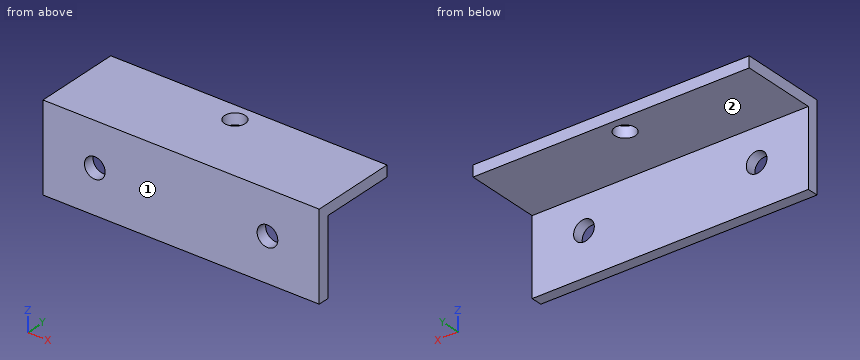
```python
from build123d import *

# Parameters (mm, degrees)
BOSS_EXTRUDE1_DEPTH = 1.6
SKETCH3_W           = 40
SKETCH3_H           = 1.6
BOSS_EXTRUDE3_DEPTH = 11
SKETCH4_R           = 1.5
CUT_EXTRUDE2_DEPTH  = 27.786563796


with BuildPart() as part:
    # Sketch1 → Boss-Extrude1 (new body)
    with BuildSketch(Plane(origin=(0, 0, 0), x_dir=(1, 0, 0), z_dir=(0, 1, 0))):
        with BuildLine():
            Line((0, 0), (0, 6.3))
            Line((0, 6.3), (-11, 6.3))
            ThreePointArc((-11, 6.3), (-12.5, 4.8), (-14, 6.3))
            Line((-14, 6.3), (-20, 6.3))
            Line((-20, 6.3), (-20, 0))
            Line((-20, 0), (0, 0))
        make_face()
        with BuildLine():
            Line((20, 6.3), (14, 6.3))
            ThreePointArc((14, 6.3), (12.5, 4.8), (11, 6.3))
            Line((11, 6.3), (0, 6.3))
            Line((0, 6.3), (0, 0))
            Line((0, 0), (20, 0))
            Line((20, 0), (20, 6.3))
        make_face()
        with BuildLine():
            ThreePointArc((11, 6.3), (12.5, 7.8), (14, 6.3))
            Line((14, 6.3), (20, 6.3))
            Line((20, 6.3), (20, 12.6))
            Line((20, 12.6), (0, 12.6))
            Line((0, 12.6), (0, 6.3))
            Line((0, 6.3), (11, 6.3))
        make_face()
        with BuildLine():
            Line((-11, 6.3), (0, 6.3))
            Line((0, 6.3), (0, 12.6))
            Line((0, 12.6), (-20, 12.6))
            Line((-20, 12.6), (-20, 6.3))
            Line((-20, 6.3), (-14, 6.3))
            ThreePointArc((-14, 6.3), (-12.5, 7.8), (-11, 6.3))
        make_face()
    extrude(amount=BOSS_EXTRUDE1_DEPTH)

    # Sketch3 → Boss-Extrude3 (add)
    with BuildSketch(Plane(origin=(0, 1.6, 0), x_dir=(1, 0, 0), z_dir=(0, 1, 0))):
        with Locations((0, 0.8)):
            Rectangle(SKETCH3_W, SKETCH3_H)
    extrude(amount=BOSS_EXTRUDE3_DEPTH)

    # Sketch4 → Cut-Extrude2 (cut, through all)
    with BuildSketch(Plane.XY):
        with Locations((0, 10)):
            Circle(SKETCH4_R)
    extrude(amount=-CUT_EXTRUDE2_DEPTH, mode=Mode.SUBTRACT)


solid = part.part
```
Input: part model. Units: mm. Frame: model coordinates. Face numbers are marked on the shaded views. A direction names the side the tool comes from. Round coordinates to 2 decimals unless told otherwise and drop trailing zeros. Loops run counter-clockwise (first coordinate to the right, second up) from the corner with the lowest first, then second, coordinate; pieces in that order, holes last. Notation, with made-up numbers: (13.25, -14.5) -> (46.25, -14.5) arc R16 cw to (46.25, -5.5) -> close; hole circle Ø7 at (19, 38). An arc over 180 degrees is marked (long way). Use one line per item in the form item = value. Start each with the question number.
Item 1: Section query C-C on x = 0. Return the cut outline in (y, z).
Item 2: Section query A-A on y = 10. Return the cut outline in (x, z), then the cut area to 3 significant figures.
Item 3: Contact query for flat-ended pins moving along their axis: pin 1 Ø5 at (x, y) = (-4.5, 4.5) entering from -Z; pin 2 Ø3 at (y, z) = (4.5, -8) entering from +X; pin 3 Ø5.5 at (x, z) = (7.5, -10) entering from +Y. Output: stop coordinate, or through.
Item 4: Set-up query: the marked faces 1 and 2. Return all of +Z, -Z, +X, -X, +Y, -Y with unobstructed straight access to the full face (end or side cutting, diameter ignored); none if empty.
Item 5: Material intervals for L1, parallel to X at y = 1.25, z = -6.3; L2, parallel to Y at x = 0, z = -0.45; L3, parallel to Z at x = -12.5, y = 1.35, sorted ascending. Write a range as from..to.
Item 6: Section query B-B on z = -6.3. Return the cut outline in (x, y), then the cut area to 3 significant figures.
Item 7: Section query D-D on z = -3. Return the cut outline in (x, y).
Ans:
q1.outline = (0, -12.6) -> (1.6, -12.6) -> (1.6, -1.6) -> (8.5, -1.6) -> (8.5, 0) -> (0, 0) -> close; (11.5, -1.6) -> (12.6, -1.6) -> (12.6, 0) -> (11.5, 0) -> close
q2.outline = (-20, -1.6) -> (-1.5, -1.6) -> (-1.5, 0) -> (-20, 0) -> close; (1.5, -1.6) -> (20, -1.6) -> (20, 0) -> (1.5, 0) -> close
q2.area = 59.2 mm^2
q3.pin_1 = -1.6
q3.pin_2 = through
q3.pin_3 = 1.6
q4.face_1 = +Z, -Z, +X, -X, -Y
q4.face_2 = -Z, +X, -X, +Y
q5.L1 = -20..-14, -11..11, 14..20
q5.L2 = 0..8.5, 11.5..12.6
q5.L3 = -12.6..-7.8, -4.8..0
q6.outline = (-20, 0) -> (-14, 0) -> (-14, 1.6) -> (-20, 1.6) -> close; (-11, 0) -> (11, 0) -> (11, 1.6) -> (-11, 1.6) -> close; (14, 0) -> (20, 0) -> (20, 1.6) -> (14, 1.6) -> close
q6.area = 54.4 mm^2
q7.outline = (-20, 0) -> (20, 0) -> (20, 1.6) -> (-20, 1.6) -> close
